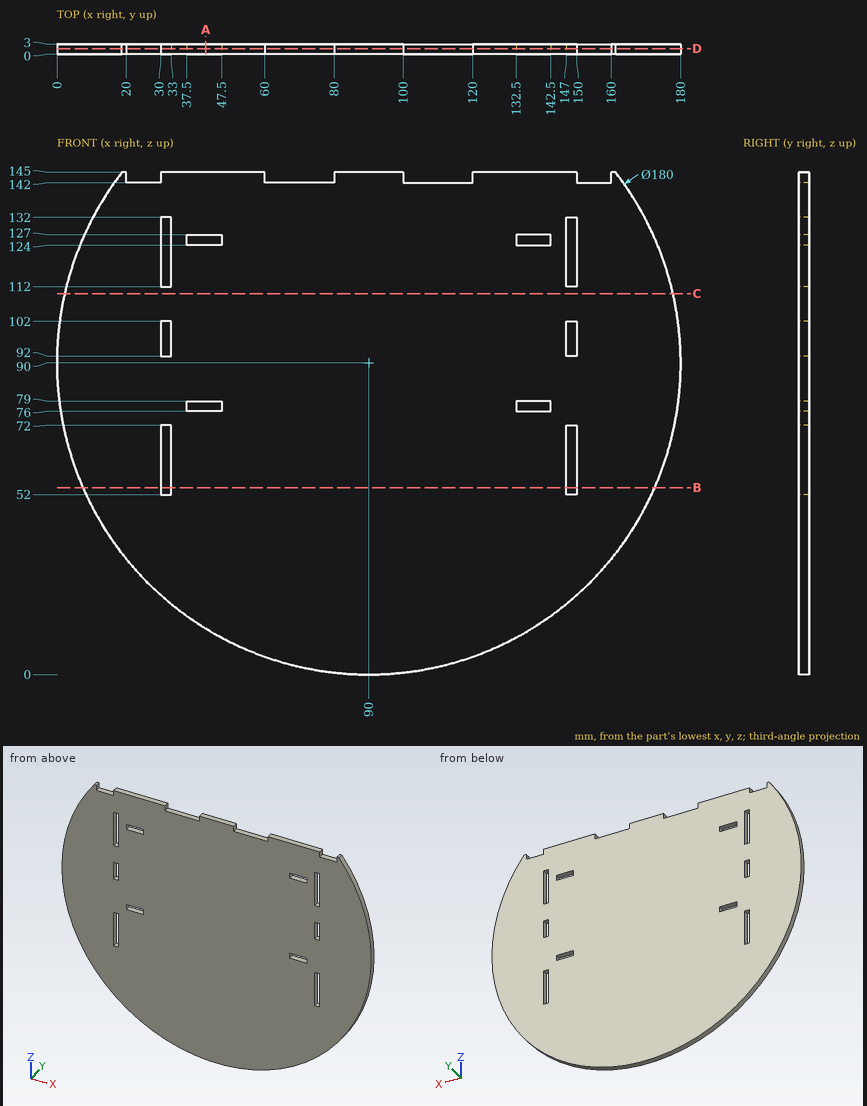
Print and shaded views of the part. All mm, measured from the part's lowest x, y and z. Give positions to 0.01 mm unless a question says otherwise; leave off trailing zeros. Write each loop counter-clockwise with the first axis right and the second up, starting at its lowest first coordinate (ties: lowest second). Pieces come first, ordered by that corner, then holes. Notation, with made-up numbers: M 51.5,62 L 57.5,62 A5 ccw 57.5,71 Z; hole C 77.25,-17 d9. An arc over 180 degrees is marked long. Use a Markdown table: item, result.
1) Drill centre lines: line 1 (Z direction, x = 135, y = 1.55); line 2 (Z direction, x = 141, y = 0.25); line 3 (X direction, y = 2.1, z = 55.5). Where is each one in solid material? Low to high. Write a range as from..to.
Responses:
| item | result |
|---|---|
| line 1 | z = 12.06..76, 79..124, 127..145 |
| line 2 | z = 15.84..76, 79..124, 127..145 |
| line 3 | x = 6.88..30, 33..147, 150..173.12 |
2) Cut at C-C (z = 110). List the corners of the cut face in (x, y).
Responses:
| item | result |
|---|---|
| outline | M 2.25,0 L 177.75,0 L 177.75,3 L 2.25,3 Z |
3) Pin check, flat tips, straight feed: pin 1 (1.5 mm diameter, centred on x = 139.5, y = 2, fed in from -Z); pin 2 (1.5 mm diameter, centred on y = 2, z = 95, fed in from +X); pin 3 (1.5 mm diameter, centred on y = 2, z = 97.5, fed in from +X). Stop position of each tip, or through.
Responses:
| item | result |
|---|---|
| pin 1 | stops at z = 14.35 |
| pin 2 | stops at x = 179.9 |
| pin 3 | stops at x = 179.75 |
4) Cut at A-A (x = 43). List the corners of the cut face in (y, z).
Responses:
| item | result |
|---|---|
| outline | M 0,13.25 L 3,13.25 L 3,76 L 0,76 Z; M 0,79 L 3,79 L 3,124 L 0,124 Z; M 0,127 L 3,127 L 3,145 L 0,145 Z |
5) Cut at D-D (y = 1.7). Give the number of separate pieces and of enclosed holes in the cut face, and give its area (3 significant figures).
Responses:
| item | result |
|---|---|
| separate pieces | 1 |
| enclosed holes | 10 |
| area | 21,400 mm2 |
6) Cut at B-B (z = 54). List the corners of the cut face in (x, y), and give its area (3 significant figures).
Responses:
| item | result |
|---|---|
| outline | M 7.51,0 L 30,0 L 30,3 L 7.51,3 Z; M 33,0 L 147,0 L 147,3 L 33,3 Z; M 150,0 L 172.49,0 L 172.49,3 L 150,3 Z |
| area | 477 mm2 |
